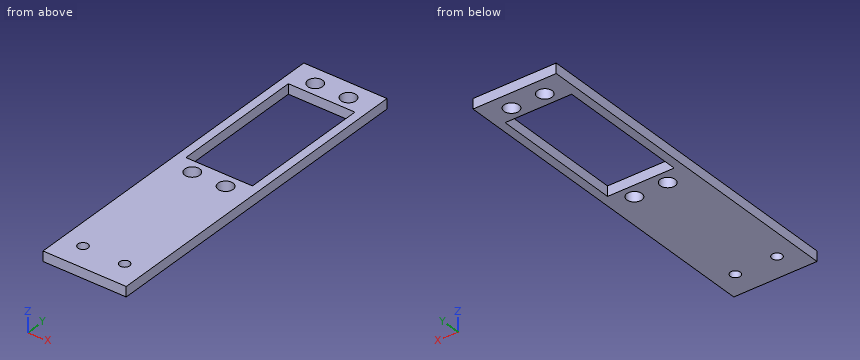
```python
from build123d import *

# Parameters (mm, degrees)
SKETCH1_W           = 25
SKETCH1_H           = 15
SKETCH1_R           = 1.5
SKETCH1_H_2         = 86.812035999
SKETCH1_R_2         = 2.25
BOSS_EXTRUDE1_DEPTH = 3


with BuildPart() as part:
    # Sketch1 → Boss-Extrude1 (new body)
    # profile 1 of 2: a face of its own
    with BuildSketch(Plane.XY):
        with Locations((12.5, 7.5)):
            Rectangle(SKETCH1_W, SKETCH1_H)
        with Locations((6.25, 7.5)):
            Circle(SKETCH1_R, mode=Mode.SUBTRACT)
        with Locations((18.75, 7.5)):
            Circle(SKETCH1_R, mode=Mode.SUBTRACT)
    # profile 2 of 2: a face of its own
    with BuildSketch(Plane.XY):
        with Locations((12.5, 58.406018)):
            Rectangle(SKETCH1_W, SKETCH1_H_2)
        with Locations((7.5, 48.53)):
            Circle(SKETCH1_R_2, mode=Mode.SUBTRACT)
        with BuildLine():
            ThreePointArc((19.75, 48.53), (17.5, 46.28), (15.25, 48.53))
            ThreePointArc((15.25, 48.53), (17.5, 50.78), (19.75, 48.53))
        make_face(mode=Mode.SUBTRACT)
        with Locations((7.5, 96.53)):
            Circle(SKETCH1_R_2, mode=Mode.SUBTRACT)
        Polygon((2.5, 52.53), (2.5, 92.53), (12.5, 92.53), (22.5, 92.53), (22.5, 52.53), (12.5, 52.53), align=None, mode=Mode.SUBTRACT)
        with Locations((17.5, 96.53)):
            Circle(SKETCH1_R_2, mode=Mode.SUBTRACT)
    extrude(amount=BOSS_EXTRUDE1_DEPTH)


solid = part.part
```
Read the model definition and answer for the solid it produces. Units are mm, in the model's axes. Coordinates: 2 decimals unless noted, no trailing zeros. Write each loop counter-clockwise with the first axis right and the second up, starting at its lowest first coordinate (ties: lowest second). Pieces come first, ordered by that corner, then holes. Notation, with made-up numbers: (1, 76) -> (19, 76) arc R16 cw to (19, 89) -> close; hole circle Ø10 at (-15, -11). An arc over 180 degrees is marked (long way). Answer as a JSON object with one key per item and string values.
Q1. Consider line 1 (Y direction, x = 18.75, z = 2.3); line 2 (Y direction, x = 10, z = 2.3); line 3 (Y direction, x = 9, z = 0.8). Determine where each line is inside the solid, lowest interval first. Write a range as [from, to].
The answers:
{"line 1": "y = [0, 6], [9, 46.66], [50.4, 52.53], [92.53, 94.66], [98.4, 101.81]", "line 2": "y = [0, 52.53], [92.53, 101.81]", "line 3": "y = [0, 46.85], [50.21, 52.53], [92.53, 94.85], [98.21, 101.81]"}
Q2. The part is cut by section D-D on y = 7.5. Give the vertices of the cut face in (x, z), then the cut area to 3 significant figures.
The answers:
{"outline": "(0, 0) -> (4.75, 0) -> (4.75, 3) -> (0, 3) -> close; (7.75, 0) -> (17.25, 0) -> (17.25, 3) -> (7.75, 3) -> close; (20.25, 0) -> (25, 0) -> (25, 3) -> (20.25, 3) -> close", "area": "57.0 mm2"}
Q3. The part is cut by section C-C on z = 2.4. Give the vertices of the cut face in (x, y).
The answers:
{"outline": "(0, 0) -> (25, 0) -> (25, 101.81) -> (0, 101.81) -> close; hole (2.5, 52.53) -> (22.5, 52.53) -> (22.5, 92.53) -> (2.5, 92.53) -> close; hole circle Ø3 at (6.25, 7.5); hole circle Ø4.5 at (7.5, 48.53); hole circle Ø4.5 at (7.5, 96.53); hole circle Ø4.5 at (17.5, 48.53); hole circle Ø4.5 at (17.5, 96.53); hole circle Ø3 at (18.75, 7.5)"}
Q4. The part is cut by section B-B on x = 3.5. Give the vertices of the cut face in (y, z), then the cut area to 3 significant figures.
The answers:
{"outline": "(0, 0) -> (52.53, 0) -> (52.53, 3) -> (0, 3) -> close; (92.53, 0) -> (101.81, 0) -> (101.81, 3) -> (92.53, 3) -> close", "area": "185 mm2"}
Q5. The part is cut by section A-A on y = 96.53. Give the vertices of the cut face in (x, z), then the cut area to 3 significant figures.
The answers:
{"outline": "(0, 0) -> (5.25, 0) -> (5.25, 3) -> (0, 3) -> close; (9.75, 0) -> (15.25, 0) -> (15.25, 3) -> (9.75, 3) -> close; (19.75, 0) -> (25, 0) -> (25, 3) -> (19.75, 3) -> close", "area": "48.0 mm2"}
